```python
from build123d import *

# Parameters (mm, degrees)
SKETCH1_R         = 11.5
EXTRUDE1_DEPTH    = 43.4
EXTRUDE2_REACH    = 58.454
CIRPATTERN1_COUNT = 12


with BuildPart() as part:
    # Sketch1 → Extrude1 (new body)
    with BuildSketch(Plane.XY):
        with BuildLine():
            ThreePointArc((6.569682115, 22.724006281), (0, 26.8), (-6.569682115, 22.724006281))
            ThreePointArc((-6.569682115, 22.724006281), (-10.625, 18.40303983), (-16.394725658, 17.051514747))
            ThreePointArc((-16.394725658, 17.051514747), (-23.209480821, 13.4), (-22.964407773, 5.672491534))
            ThreePointArc((-22.964407773, 5.672491534), (-21.25, 0), (-22.964407773, -5.672491534))
            ThreePointArc((-22.964407773, -5.672491534), (-23.209480821, -13.4), (-16.394725658, -17.051514747))
            ThreePointArc((-16.394725658, -17.051514747), (-10.625, -18.40303983), (-6.569682115, -22.724006281))
            ThreePointArc((-6.569682115, -22.724006281), (0, -26.8), (6.569682115, -22.724006281))
            ThreePointArc((6.569682115, -22.724006281), (10.625, -18.40303983), (16.394725658, -17.051514747))
            ThreePointArc((16.394725658, -17.051514747), (23.209480821, -13.4), (22.964407773, -5.672491534))
            ThreePointArc((22.964407773, -5.672491534), (21.25, 0), (22.964407773, 5.672491534))
            ThreePointArc((22.964407773, 5.672491534), (23.209480821, 13.4), (16.394725658, 17.051514747))
            ThreePointArc((16.394725658, 17.051514747), (10.625, 18.40303983), (6.569682115, 22.724006281))
        make_face()
        Circle(SKETCH1_R, mode=Mode.SUBTRACT)
    extrude(amount=EXTRUDE1_DEPTH)

    # Sketch4 → Cut-Revolve1 (revolve, cut)
    with BuildSketch(Plane(origin=(0, 0, 0), x_dir=(0, 0, -1), z_dir=(1, 0, 0)), mode=Mode.PRIVATE) as cut_revolve1_sk:
        Polygon((0, 0), (-43.4, 0), (-43.4, 12.05), (-42.9, 11.55), (-0.5, 11.55), (0, 12.05), align=None)
    revolve(cut_revolve1_sk.sketch.rotate(Axis((0, 0, 0), (0, 0, 1)), 90), axis=Axis((0, 0, 0), (0, 0, 1)), mode=Mode.SUBTRACT)

    # Sketch2 → Extrude2 (cut, up to next)
    with BuildSketch(Plane(origin=(0, 0, 0), x_dir=(-1, 0, 0), z_dir=(0, 0, -1)), mode=Mode.PRIVATE) as extrude2_sk1:
        with BuildLine():
            ThreePointArc((1.54, 13.864735843), (0, 13.95), (-1.54, 13.864735843))
            ThreePointArc((-1.54, 13.864735843), (-2.042378597, 12.605566852), (-2.4, 11.297898035))
            ThreePointArc((-2.4, 11.297898035), (0, 11.55), (2.4, 11.297898035))
            ThreePointArc((2.4, 11.297898035), (2.042378597, 12.605566852), (1.54, 13.864735843))
        make_face()
    extrude2_tool1 = extrude(extrude2_sk1.sketch, amount=-EXTRUDE2_REACH, mode=Mode.PRIVATE) & part.part
    extrude2 = extrude2_tool1.solids().sort_by_distance((0, 12.606446, 0))[0]
    add(extrude2, mode=Mode.SUBTRACT)

    # CirPattern1: Extrude2 ×12 about axis
    cirpattern1_axis = Axis((0, 0, 0), (0, 0, 1))
    for i in range(1, CIRPATTERN1_COUNT):
        add(extrude2.rotate(cirpattern1_axis, i * 360 / CIRPATTERN1_COUNT), mode=Mode.SUBTRACT)


solid = part.part
```
Here's how the part is built. I have some questions about the finished solid (model axes, mm). A direction names the side the tool comes from. Give positions to 0.01 mm unless a question says otherwise; leave off trailing zeros. Loops run counter-clockwise (first coordinate to the right, second up) from the corner with the lowest first, then second, coordinate; pieces in that order, holes last. Notation, with made-up numbers: (66, 30.5) -> (115, 30.5) arc R16 ccw to (115, 38.5) -> close; hole circle Ø8 at (5, -25.5). An arc over 180 degrees is marked (long way). Use one line per item in the form item = value. Start each with the question number.
1) Please list where these lines run through material, in increasing order: line 1 along Y through (x, z) = (-15, 30); line 2 along Y through (x, z) = (-12, 14); line 3 along X through (y, z) = (10.5, 30).
2) Thinking about a two-plate mould opening in Y: for faces 4 (the face through (-13.95, -0.02, 21.4)), 5 (the face through (10.7, 18.36, 21.4)), 6 (the face through (10, -12, 0)), which applies, +Y half, -Y half, draft (parallel to the pull), parting line (faces both ways), or undercut?
3) Imagine slicing it at A-A (x = 19). Please give me the cut outline in (y, z), then the cut area to 3 significant figures.
4) Imagine slicing it at B-B (y = -15). Please give me the cut outline in (x, z).
5) Which directions (+Z, -Z, +X, -X, +Y, -Y) give clear straight access to the entire face, cutting with the end or side of a thin tool? Please do faces 1 (the face through (-8.34, 8.35, 0.25)), 2 (the face through (-6.96, -12.09, 21.4)), 3 (the face through (-21.25, 0.08, 21.4)).
6) For P1, Ø1, axis at y = -6, z = 7.5, coming from the +X side; P2, Ø5, axis at x = -3, z = 10, coming from the -Y side; P3, Ø8, axis at y = -17.5, z = 37, coming from the +X side, each with a flat end and sliding along its axis, tell me the tip position at first contact or that it passes through.
Check values:
q1.line_1 = -17.06 to 17.06
q1.line_2 = -17.74 to -7.11, -4.6 to -2.23, 2.23 to 4.6, 7.11 to 17.74
q1.line_3 = -24.15 to -8.18, 8.18 to 24.15
q2.face_4 = undercut
q2.face_5 = +Y half
q2.face_6 = draft
q3.outline = (-16.75, 0) -> (16.75, 0) -> (16.75, 43.4) -> (-16.75, 43.4) -> close
q3.area = 1,450 mm^2
q4.outline = (-21.96, 0) -> (21.96, 0) -> (21.96, 43.4) -> (-21.96, 43.4) -> close
q5.face_1 = -Z
q5.face_2 = +Z, -Z
q5.face_3 = +Z, -Z, -X
q6.P1 = 23.44
q6.P2 = -26.78
q6.P3 = 23.15
